Check sheet for the modelled part. Datum: model origin and axes. Units: mm. Face numbers are marked on the shaded views. A direction names the side the tool comes from. Round coordinates to 2 decimals unless told otherwise and drop trailing zeros. Order: outer loops, then holes, each group sorted by start corner. A loop starts at its lowest first (then second) coordinate and runs counter-clockwise, first axis right, second up. Notation, with made-up numbers: (63.25, -4) -> (96.25, -4) arc R7 ccw to (96.25, 0) -> close; hole circle Ø5 at (9, 40). An arc over 180 degrees is marked (long way). Answer in a Markdown table with one row per item.
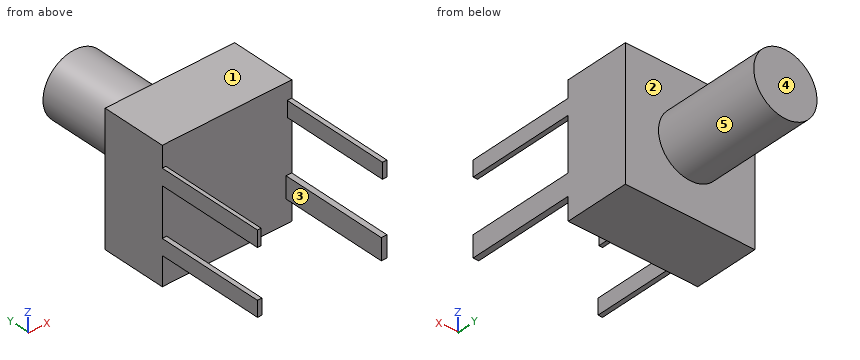
```python
from build123d import *

# Parameters (mm, degrees)
SKETCH1_W           = 6
SKETCH1_H           = 6
BOSS_EXTRUDE1_DEPTH = 3
SKETCH2_R           = 1.46607231
BOSS_EXTRUDE2_DEPTH = 5
SKETCH3_W           = 0.169867938
SKETCH3_H           = 0.743920428
SKETCH3_W_2         = 0.207603032
SKETCH3_H_2         = 0.722357517
SKETCH3_W_3         = 0.261510309
SKETCH3_H_3         = 0.986503176
BOSS_EXTRUDE3_DEPTH = 5


with BuildPart() as part:
    # Sketch1 → Boss-Extrude1 (new body)
    with BuildSketch(Plane(origin=(0, 0, 0), x_dir=(1, 0, 0), z_dir=(0, 1, 0))):
        with Locations((3, -3)):
            Rectangle(SKETCH1_W, SKETCH1_H)
    extrude(amount=BOSS_EXTRUDE1_DEPTH)

    # Sketch2 → Boss-Extrude2 (add)
    with BuildSketch(Plane(origin=(0, 3, 0), x_dir=(1, 0, 0), z_dir=(0, 1, 0))):
        with Locations(Location((3, -3, 0), (0, 0, 270))):
            Circle(SKETCH2_R)
    extrude(amount=BOSS_EXTRUDE2_DEPTH)

    # Sketch3 → Boss-Extrude3 (add)
    with BuildSketch(Plane(origin=(0, 0, 0), x_dir=(-1, 0, 0), z_dir=(0, -1, 0))):
        with Locations((-0.084933969, -4.657648779)):
            Rectangle(SKETCH3_W, SKETCH3_H)
        with Locations((-0.103801516, -1.687357796)):
            Rectangle(SKETCH3_W_2, SKETCH3_H_2)
        with Locations((-5.896198484, -4.857105706)):
            Rectangle(SKETCH3_W_2, SKETCH3_H_2)
        with Locations((-5.869244846, -1.555284966)):
            Rectangle(SKETCH3_W_3, SKETCH3_H_3)
    extrude(amount=BOSS_EXTRUDE3_DEPTH)


solid = part.part
```
(1) Section check B-B on x = 3. Record the boundary of the cut face in (y, z), plus the area to 3 significant figures.
Solutions:
| item | result |
|---|---|
| outline | (0, 0) -> (3, 0) -> (3, 1.53) -> (8, 1.53) -> (8, 4.47) -> (3, 4.47) -> (3, 6) -> (0, 6) -> close |
| area | 32.7 mm^2 |
(2) Draft check along X on the marked faces 3, 4 and 5. Enter one of: pulls with the +X half, pulls with the -X half, needs draft (parallel to the pull), parting line crosses it, or undercut.
Solutions:
| item | result |
|---|---|
| face 3 | undercut |
| face 4 | needs draft |
| face 5 | parting line crosses it |
(3) Depth check by flat-ended pin: pin 1 Ø3 at (x, y) = (3, 2.5) entering from -Z; pin 2 Ø2 at (x, y) = (2.5, 4.5) entering from +Z; pin 3 Ø3 at (x, y) = (1.5, 5) entering from -Z; pin 4 Ø3 at (x, z) = (2, 2.5) entering from -Y. Enter the tip coordinate at first touch or a pass-through.
Solutions:
| item | result |
|---|---|
| pin 1 | z = 0 |
| pin 2 | z = 4.47 |
| pin 3 | z = 1.53 |
| pin 4 | y = 0 |
(4) Scan lines: probe 1 along X at (y, z) = (-2.5, 1.4); probe 2 along Y at (x, z) = (5.5, 0.5); probe 3 along Y at (x, z) = (3.25, 3.8). Record each from-to range of solid material in increasing order. Write a range as from..to.
Solutions:
| item | result |
|---|---|
| probe 1 | 0..0.21, 5.74..6 |
| probe 2 | 0..3 |
| probe 3 | 0..8 |
(5) Section check C-C on z = 3. Record the boundary of the cut face in (x, y).
Solutions:
| item | result |
|---|---|
| outline | (0, 0) -> (6, 0) -> (6, 3) -> (4.47, 3) -> (4.47, 8) -> (1.53, 8) -> (1.53, 3) -> (0, 3) -> close |
(6) Tool access check on the marked faces 1 and 2. Record the directions out of +Z, -Z, +X, -X, +Y, -Y that give a thin tool (end or side, any length) a straight path to the whole face; none if there is none.
Solutions:
| item | result |
|---|---|
| face 1 | +Z, +X, -X, +Y, -Y |
| face 2 | +Y |
(7) Section check A-A on y = -3.5. Record the boundary of the cut face in (x, z), plus the area to 3 significant figures.
Solutions:
| item | result |
|---|---|
| outline | (0, 1.33) -> (0.21, 1.33) -> (0.21, 2.05) -> (0, 2.05) -> close; (0, 4.29) -> (0.17, 4.29) -> (0.17, 5.03) -> (0, 5.03) -> close; (5.74, 1.06) -> (6, 1.06) -> (6, 2.05) -> (5.74, 2.05) -> close; (5.79, 4.5) -> (6, 4.5) -> (6, 5.22) -> (5.79, 5.22) -> close |
| area | 0.684 mm^2 |
(8) Section check D-D on y = 5. Record the boundary of the cut face in (x, z), plus the area to 3 significant figures.
Solutions:
| item | result |
|---|---|
| outline | circle Ø2.93 at (3, 3) |
| area | 6.75 mm^2 |
